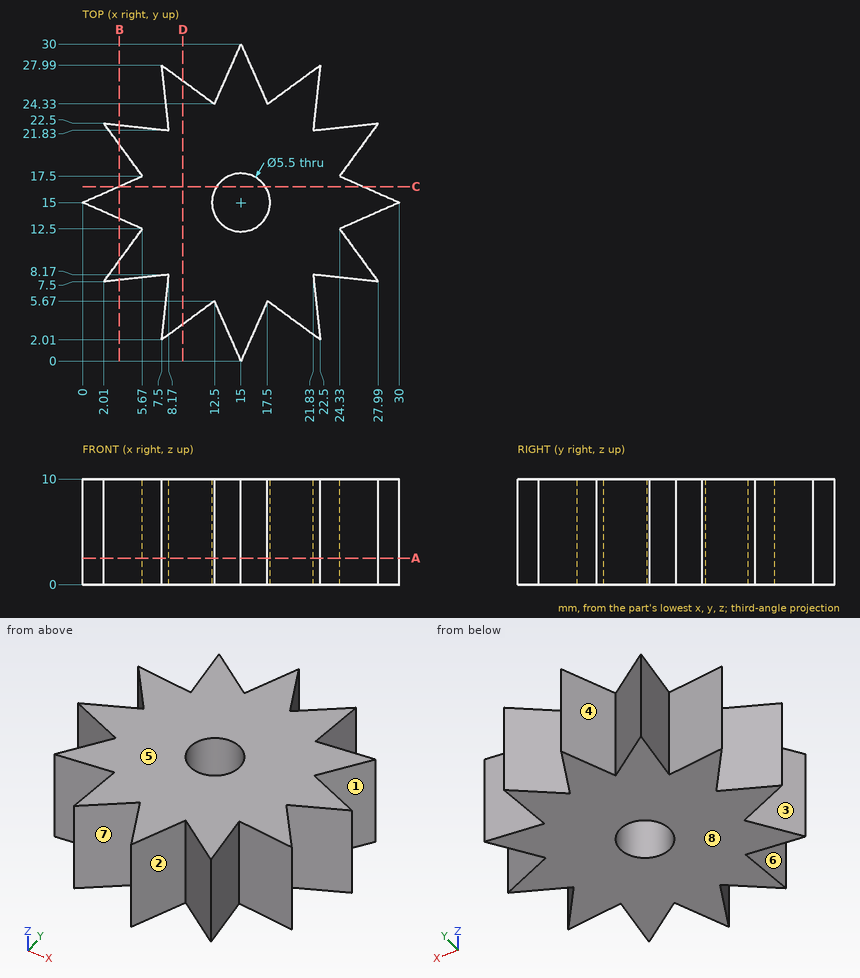
Answer from the drawing. Dimensions are ordinates in mm from the lowest x, y and z of the part. A direction names the side the tool comes from. Round coordinates to 2 decimals unless told otherwise and drop trailing zeros. Write each loop counter-clockwise with the first axis right and the second up, starting at its lowest first coordinate (ties: lowest second). Pieces come first, ordered by that corner, then holes. Notation, with made-up numbers: (65, 0.25) - (70, 0.25) arc R22 ccw to (70, 19.25) - close; hole circle Ø4 at (25.5, 18). An arc over 180 degrees is marked (long way). Use a Markdown table: item, result.
(1) The mould has two halves that part along Y. Classify the marked faces 6, 7 and 8: released by +Y, released by -Y, zero draft, split by the parting line, or undercut.
Reported:
| item | result |
|---|---|
| face 6 | undercut |
| face 7 | released by -Y |
| face 8 | zero draft |
(2) Which of the six approach directions +Z, -Z, +X, -X, +Y, -Y give full straight-line access (tool end or side, diameter ignored) to the marked faces 1, 2, 3, 4 and 5?
Reported:
| item | result |
|---|---|
| face 1 | +Z, -Z, +X |
| face 2 | +Z, -Z, -Y |
| face 3 | +Z, -Z, -X |
| face 4 | +Z, -Z, +Y |
| face 5 | +Z, +X, -X, +Y, -Y |
(3) Straight lines are drawn through the part: line 1 along X through (y, z) = (2.5, 7) (1 decimal); line 2 along Y through (x, z) = (5.5, 5.5) (1 decimal); line 3 along Y through (x, z) = (26.5, 6.25) (1 decimal). For each, find the intervals that lie inside material, in ascending order. Write a range as [from, to].
Reported:
| item | result |
|---|---|
| line 1 | [7.6, 8.2], [13.9, 16.1], [21.8, 22.4] |
| line 2 | [7.9, 12.3], [12.6, 17.4], [17.7, 22.1] |
| line 3 | [7.7, 9.5], [13.5, 16.5], [20.5, 22.3] |
(4) Each of these flat-tipped pins is pushed along its axis until it touches: pin 1 Ø1 at (y, z) = (8.5, 4.5) entering from +X (1 decimal); pin 2 Ø6 at (y, z) = (7.5, 8.5) entering from -X; pin 3 Ø1 at (y, z) = (14, 2) entering from -X (1 decimal). Where does it stop, or does it pass through?
Reported:
| item | result |
|---|---|
| pin 1 | x = 27.6 |
| pin 2 | x = 2.01 |
| pin 3 | x = 1.1 |
(5) The part is cut by section D-D (x = 9.5). Write down the section's boundary in (y, z).
Reported:
| item | result |
|---|---|
| outline | (3.47, 0) - (26.53, 0) - (26.53, 10) - (3.47, 10) - close |
(6) The part is cut by section B-B (x = 3.5). Write down the section's boundary in (y, z).
Reported:
| item | result |
|---|---|
| outline | (7.66, 0) - (9.54, 0) - (9.54, 10) - (7.66, 10) - close; (13.46, 0) - (16.54, 0) - (16.54, 10) - (13.46, 10) - close; (20.46, 0) - (22.34, 0) - (22.34, 10) - (20.46, 10) - close |
(7) The part is cut by section C-C (y = 16.5). Write down the section's boundary in (x, z) (1 decimal).
Reported:
| item | result |
|---|---|
| outline | (3.4, 0) - (12.7, 0) - (12.7, 10) - (3.4, 10) - close; (17.3, 0) - (26.6, 0) - (26.6, 10) - (17.3, 10) - close |
(8) The part is cut by section A-A (z = 2.5). Write down the section's boundary in (x, y).
Reported:
| item | result |
|---|---|
| outline | (0, 15) - (5.67, 12.5) - (2.01, 7.5) - (8.17, 8.17) - (7.5, 2.01) - (12.5, 5.67) - (15, 0) - (17.5, 5.67) - (22.5, 2.01) - (21.83, 8.17) - (27.99, 7.5) - (24.33, 12.5) - (30, 15) - (24.33, 17.5) - (27.99, 22.5) - (21.83, 21.83) - (22.5, 27.99) - (17.5, 24.33) - (15, 30) - (12.5, 24.33) - (7.5, 27.99) - (8.17, 21.83) - (2.01, 22.5) - (5.67, 17.5) - close; hole circle Ø5.5 at (15, 15) |
